from build123d import *

# Parameters (mm, degrees)
F0_W     = 75
F0_H     = 75
F1_DEPTH = 75
F2_T     = -2
F4_DEPTH = 146.3
F6_DEPTH = 84.9
F8_DEPTH = 25


with BuildPart() as f1:
    # F0 (on Front) → F1 (new body)
    with BuildSketch(Plane.XZ):
        with Locations((-2.307421, 2.156376)):
            Rectangle(F0_W, F0_H)
    extrude(amount=-F1_DEPTH)

    # F2
    f2_openings = [f1.faces().sort_by_distance(p)[0] for p in [
        (-2.307421, 0, 2.156376),
    ]]
    offset(amount=F2_T, openings=f2_openings)

    # F3 (on face) → F4 (cut)
    with BuildSketch(Plane(origin=(0, 0, -35.343624), x_dir=(1, 0, 0), z_dir=(0, 0, -1))):
        Polygon((-20.990076, -20.543478), (-25.009453, -54.782614), (-20.990076, -59.099723), align=None)
        Polygon((6.550096, -54.782614), (-15.779775, -21.734407), (-13.993384, -47.488187), align=None)
        Polygon((10.420605, -33.048205), (0, -11.164933), (9.080812, -51.507566), (27.54017, -26.051514), align=None)
        Polygon((23.371927, -63.863426), (-13.100189, -54.782614), (-12.35586, -60.886107), align=None)
        Polygon((-4.912571, -13.397922), (-15.779775, -14.291116), (2.988963, -42.068847), align=None)
        Polygon((-32.006145, -54.782614), (-20.990076, -9.676277), (-32.006145, -21.734407), align=None)
        Polygon((29.545442, -49.04395), (27.218709, -41.974761), (12.761539, -57.036284), align=None)
        Polygon((24.409195, -16.750237), (9.080812, -13.030036), (20.074258, -24.837809), align=None)
    extrude(amount=-F4_DEPTH, mode=Mode.SUBTRACT)

    # F5 (on face) → F6 (cut)
    with BuildSketch(Plane.YZ.offset(35.192579)):
        Polygon((15.842715, -16.520021), (13.993383, -28.284499), (59.546318, -13.695653), align=None)
        Polygon((22.829311, 15.588589), (18.369781, -11.168586), (31.302415, 6.818181), align=None)
        Polygon((48.991881, 15.737241), (24.761772, -11.168586), (40.072825, -9.087472), align=None)
        Polygon((24.761772, 35.430476), (23.225486, 23.14827), (36.825874, 13.36948), align=None)
        Polygon((30.14504, 34.565531), (38.275514, 26.435059), (59.546318, 17.439637), align=None)
        Polygon((59.546318, 9.522333), (45.022078, -6.60581), (56.95831, -2.800056), align=None)
        Polygon((45.022078, 19.038399), (38.275514, 23.14827), (42.701558, 15.054593), align=None)
    extrude(amount=-F6_DEPTH, mode=Mode.SUBTRACT)

    # F7 (on face) → F8 (cut)
    with BuildSketch(Plane(origin=(0, 75, 0), x_dir=(-1, 0, 0), z_dir=(0, 1, 0))):
        Polygon((-20.296717, -3.729921), (3.701246, 27.96888), (-3.999593, 26.536167), align=None)
        Polygon((7.46212, 25.461631), (9.253013, 24.208006), (13.730245, -11.43076), (13.730245, 25.461631), align=None)
        Polygon((9.253013, -9.287988), (3.701246, 16.865345), (-16.356753, -12.505296), align=None)
        Polygon((-23.878502, -11.43076), (-23.878502, 12.567203), (-28.534822, -17.340705), (-2.925058, -17.340705), align=None)
        Polygon((30.441476, 4.064158), (14.80478, 27.96888), (26.445584, 3.075472), (18.446537, -11.779902), align=None)
        Polygon((19.680761, 2.233784), (16.774762, 8.44815), (18.227762, -0.464643), align=None)
        Polygon((0, -23.215262), (26.803762, -19.847956), (11.629337, -17.777083), align=None)
        Polygon((-9.792007, 24.208006), (-21.192163, 33.162467), (-18.604818, 12.567203), align=None)
    extrude(amount=-F8_DEPTH, mode=Mode.SUBTRACT)


solid = f1.part
Geometry check sheet. Reference: the model listing, model coordinates, mm. A direction names the side the tool comes from. Coordinates: 2 decimals unless noted, no trailing zeros. Order: outer loops, then holes, each group sorted by start corner. A loop starts at its lowest first (then second) coordinate and runs counter-clockwise, first axis right, second up. Notation, with made-up numbers: (52, 85) -> (64, 85) arc R8 cw to (64, 90) -> close; hole circle Ø9 at (-17.5, 43). An arc over 180 degrees is marked (long way). Use a Markdown table: item, result. Add a question column.
1. Material ranges on L1, parallel to X at y = 60.5, z = 2; L2, parallel to Z at x = 2, y = 54; L3, parallel to Y at x = 21, z = -5, recorded low to high.
2. Set-up check for faces 1 (the face through (-3, 36, -33.344)), 2 (the face through (34.21, 44.47, 3.15)), 3 (the face through (-3.865, 51.084, -34.358)): record each of +Z, -Z, +X, -X, +Y, -Y from which the full face is reachable in a straight line by a thin tool's end or side.
3. Cross-section at B-B (y = 29). Give the number of separate pieces and of enclosed holes in the cut face, and give its area (3 significant figures).
4. Go/stop test with a flat-tipped pin: pin 1 Ø3 at (x, z) = (-8, 1.5) entering from -Y. Record where the tip stops, or that it passes through.
5. Mould release check, pull along X, two halves, no side actions. Record for faces 4 (the face through (35.193, 37, 10)), 5 (the face through (8.466, 74.014, 11.898)), 6 (the face through (-38.793, 27.125, 11.142)): pulls with the +X half, pulls with the -X half, needs draft (parallel to the pull), parting line crosses it, or undercut.
6. Cross-section at A-A (y = 65). Enter the section's corners in (x, z).
Filled sheet:
| question | item | result |
|---|---|---|
| 1 | L1 | -39.81 to -37.81, 33.19 to 35.19 |
| 1 | L2 | -35.34 to -33.34, 37.66 to 39.66 |
| 1 | L3 | 73 to 75 |
| 2 | face 1 | -Y |
| 2 | face 2 | +X, -X |
| 2 | face 3 | +Z, -Z |
| 3 | separate pieces | 20 |
| 3 | enclosed holes | 0 |
| 3 | area | 373 mm2 |
| 4 | pin 1 | y = 73 |
| 5 | face 4 | pulls with the +X half |
| 5 | face 5 | undercut |
| 5 | face 6 | needs draft |
| 6 | outline | (-39.81, -35.34) -> (35.19, -35.34) -> (35.19, 39.66) -> (-39.81, 39.66) -> close; hole (-37.81, -33.34) -> (33.19, -33.34) -> (33.19, 37.66) -> (-37.81, 37.66) -> close |
